Can you work these out from the drawing? Everything is in mm from the part's minimum corner. Round coordinates to 2 decimals unless told otherwise and drop trailing zeros. Write each loop counter-clockwise with the first axis right and the second up, starting at its lowest first coordinate (ties: lowest second). Pieces come first, ordered by that corner, then holes. Notation, with made-up numbers: (-31, 24.25) -> (-21, 24.25) arc R28 ccw to (-21, 60.25) -> close; hole circle Ø7 at (9.5, 1.25). An arc over 180 degrees is marked (long way). Put each result on its own line as item: value. Start each with the question number.
1. For pin 1 (2.5 mm diameter, centred on x = 14.5, z = 19, fed in from +Y); pin 2 (1 mm diameter, centred on x = 11.5, y = 3, fed in from -Z), each with a flat end and sliding along its axis, tell me the tip position at first contact or that it passes through.
2. We'd pull the mould along Z, two halves only. Please class the marked faces 1, 2 and 3: +Z half, -Z half, draft (parallel to the pull), parting line (faces both ways), or undercut.
3. Suppose I cut it at B-B (x = 23). Please give me the cut outline in (y, z), then the cut area to 3 significant figures.
4. I need wall thicknesses on probe 1 along Z at (x, y) = (23.5, 3.4); probe 2 along Z at (x, y) = (17.5, 4.55); probe 3 along Z at (x, y) = (8, 4.6). Which ranges of each line are inside material? Lowest first, please. Write a range as from..to.
5. Suppose I cut it at D-D (x = 3.5). Please give me the cut outline in (y, z).
6. Suppose I cut it at A-A (z = 19). Please give me the cut outline in (x, y).
7. Suppose I cut it at C-C (y = 3.25). Please give me the cut outline in (x, z).
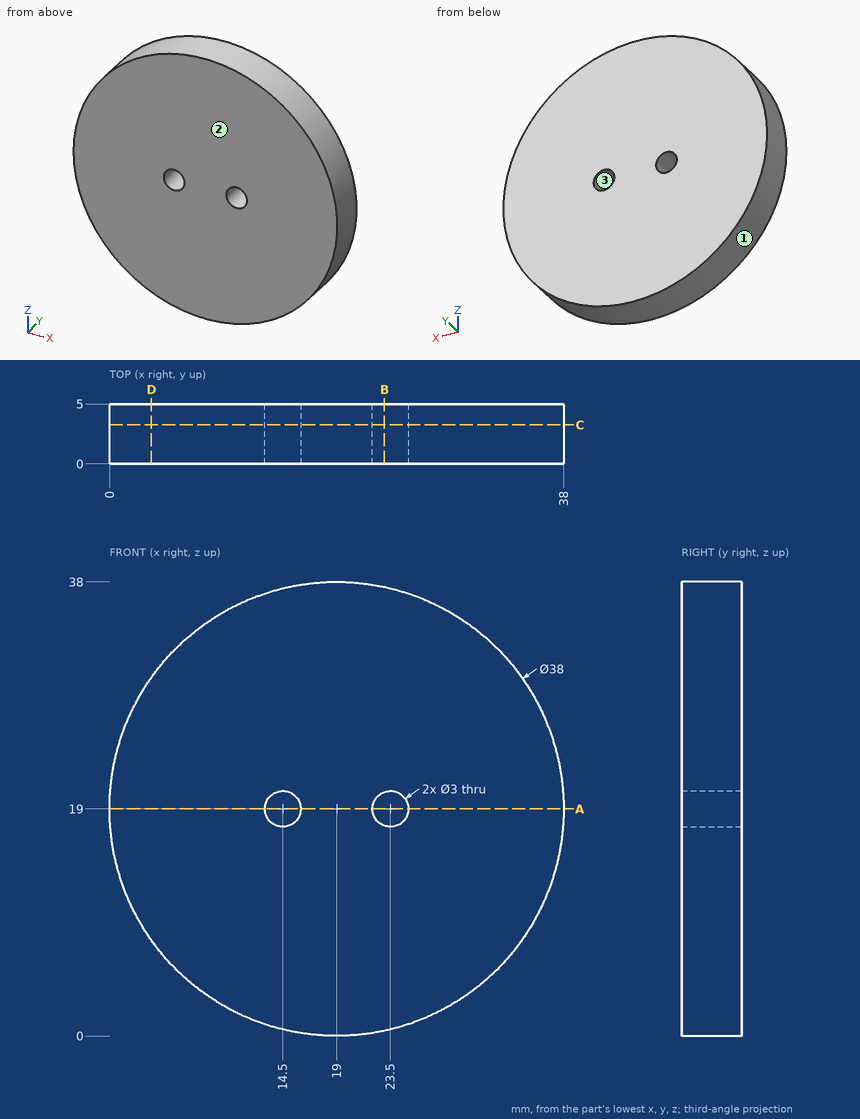
Verdict:
1. pin 1: passes through
1. pin 2: stops at z = 1.34
2. face 1: parting line
2. face 2: draft
2. face 3: undercut
3. outline: (0, 0.43) -> (5, 0.43) -> (5, 17.59) -> (0, 17.59) -> close; (0, 20.41) -> (5, 20.41) -> (5, 37.57) -> (0, 37.57) -> close
3. area: 172 mm^2
4. probe 1: z = 0.54..17.5, 20.5..37.46
4. probe 2: z = 0.06..37.94
4. probe 3: z = 3.51..34.49
5. outline: (0, 8.01) -> (5, 8.01) -> (5, 29.99) -> (0, 29.99) -> close
6. outline: (0, 0) -> (13, 0) -> (13, 5) -> (0, 5) -> close; (16, 0) -> (22, 0) -> (22, 5) -> (16, 5) -> close; (25, 0) -> (38, 0) -> (38, 5) -> (25, 5) -> close
7. outline: circle Ø38 at (19, 19); hole circle Ø3 at (14.5, 19); hole circle Ø3 at (23.5, 19)
